Print and shaded views of the part. All mm, measured from the part's lowest x, y and z. A direction names the side the tool comes from. Give positions to 0.01 mm unless a question says otherwise; leave off trailing zeros. Order: outer loops, then holes, each group sorted by start corner. A loop starts at its lowest first (then second) coordinate and runs counter-clockwise, first axis right, second up. Notation, with made-up numbers: (23.5, -16.75) - (27.5, -16.75) arc R8 ccw to (27.5, -7.75) - close; hole circle Ø5 at (14, 78). An arc over 180 degrees is marked (long way). Answer in a Markdown table with one row per item.
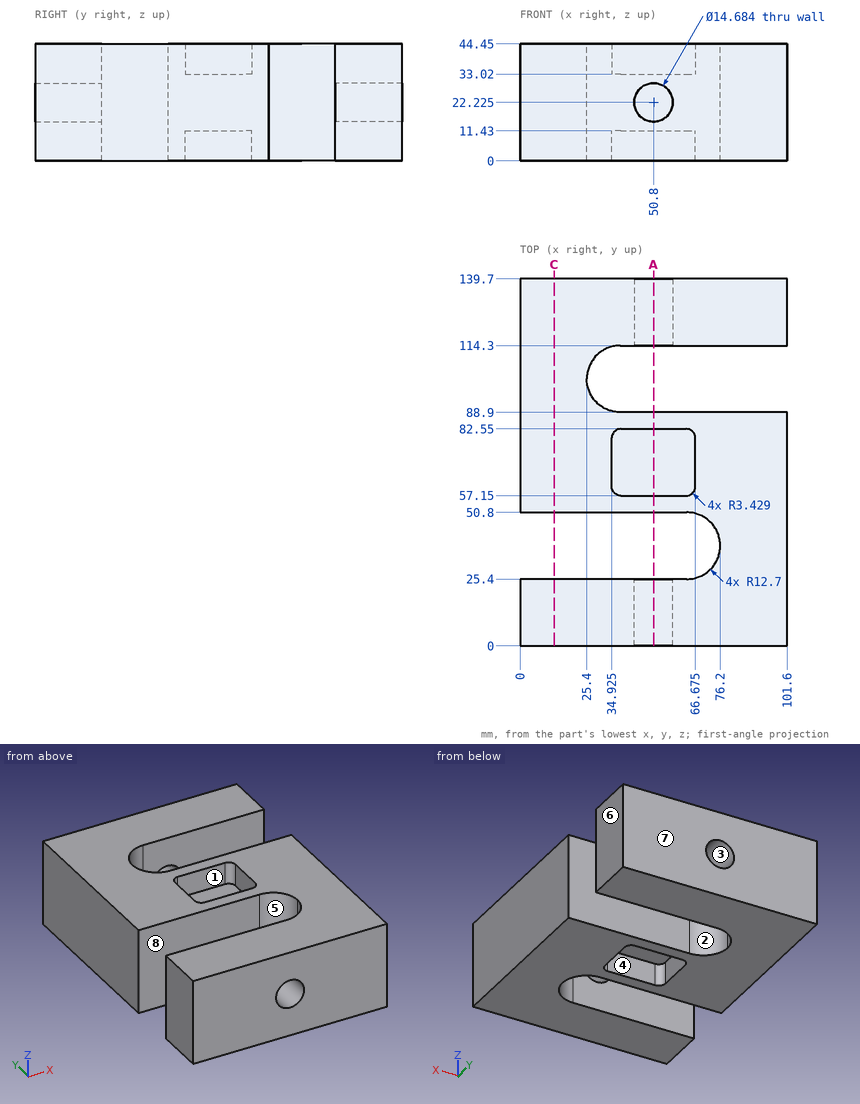
1. Which spindle directions (+Z, -Z, +X, -X, +Y, -Y) get a long thin tool onto all of the face, cutting with end or side? Do the marked faces 1, 2, 3, 4 and 5. Say none if no direction does.
Check result:
| item | result |
|---|---|
| face 1 | +Z |
| face 2 | +Z, -Z, +X |
| face 3 | +Y |
| face 4 | -Z |
| face 5 | +Z, -Z, -X |
2. Cut at A-A on x = 50.8. Write the cut outline in (y, z).
Check result:
| item | result |
|---|---|
| outline | (0, 0) - (25.4, 0) - (25.4, 14.88) - (0, 14.88) - close; (0, 29.57) - (25.4, 29.57) - (25.4, 44.45) - (0, 44.45) - close; (50.8, 0) - (57.15, 0) - (57.15, 11.43) - (82.55, 11.43) - (82.55, 0) - (88.9, 0) - (88.9, 44.45) - (82.55, 44.45) - (82.55, 33.02) - (57.15, 33.02) - (57.15, 44.45) - (50.8, 44.45) - close; (114.3, 0) - (139.7, 0) - (139.7, 14.88) - (114.3, 14.88) - close; (114.3, 29.57) - (139.7, 29.57) - (139.7, 44.45) - (114.3, 44.45) - close |
3. Two-plate mould, pull along Y, no slides. Class the marked faces 6, 7 and 8: +Y half, -Y half, draft (parallel to the pull), parting line (faces both ways), or undercut.
Check result:
| item | result |
|---|---|
| face 6 | draft |
| face 7 | +Y half |
| face 8 | undercut |
4. Cut at C-C on x = 13. Write the cut outline in (y, z), and give its area (3 significant figures).
Check result:
| item | result |
|---|---|
| outline | (0, 0) - (25.4, 0) - (25.4, 44.45) - (0, 44.45) - close; (50.8, 0) - (139.7, 0) - (139.7, 44.45) - (50.8, 44.45) - close |
| area | 5,080 mm² |
5. Drop flat-ended pins along their axis: P1, Ø9, axis at y = 67, z = 6, coming from the -X side; P2, Ø11.5, axis at x = 50.8, z = 22.225, coming from the -Y side; P3, Ø7.5, axis at x = 47.5, y = 63.5, coming from the +Z side; P4, Ø7.5, axis at x = 45, y = 67, coming from the -Z side. Give the stop position or say it passes through.
Check result:
| item | result |
|---|---|
| P1 | stops at x = 0 |
| P2 | stops at y = 50.8 |
| P3 | stops at z = 33.02 |
| P4 | stops at z = 11.43 |
6. Probe line 1 (Y direction, x = 55.5, z = 14); line 2 (Y direction, x = 83, z = 18); line 3 (Y direction, x = 63.5, z = 11). List the from-to ranges inside material, lowest first.
Check result:
| item | result |
|---|---|
| line 1 | y = 0 to 25.4, 50.8 to 88.9, 114.3 to 139.7 |
| line 2 | y = 0 to 88.9, 114.3 to 139.7 |
| line 3 | y = 0 to 25.4, 50.8 to 57.16, 82.54 to 88.9, 114.3 to 139.7 |
